CAD build for the part. Positions are in the model's coordinates, mm. A direction names the side the tool comes from. Round coordinates to 2 decimals unless told otherwise and drop trailing zeros. Order: outer loops, then holes, each group sorted by start corner. A loop starts at its lowest first (then second) coordinate and runs counter-clockwise, first axis right, second up. Notation, with made-up numbers: M 53,52.25 L 67,52.25 A31 ccw 67,91.25 Z; hole C 69,14 d8. An arc over 180 degrees is marked long. Put each result on its own line as item: value.
```python
from build123d import *

# Parameters (mm, degrees)
BOSS_EXTRUDE1_DEPTH = 6
SKETCH4_W           = 3
SKETCH4_H           = 3
CUT_EXTRUDE2_DEPTH  = 32
SKETCH5_R           = 1.75
CUT_EXTRUDE3_DEPTH  = 10


with BuildPart() as part:
    # Sketch1 → Boss-Extrude1 (new body)
    with BuildSketch(Plane(origin=(0, 0, 0), x_dir=(0, 1, 0), z_dir=(0, 0, 1))):
        with BuildLine():
            Line((-92.5, -9.5), (-94.5, -9.5))
            ThreePointArc((-94.5, -9.5), (-95.207106781, -9.792893219), (-95.5, -10.5))
            Line((-95.5, -10.5), (-95.5, -27.5))
            Line((-95.5, -27.5), (-95.5, -37.5))
            Line((-95.5, -37.5), (-99, -37.5))
            ThreePointArc((-99, -37.5), (-99.459572515, -37.196959649), (-99.362068966, -36.655172414))
            ThreePointArc((-99.362068966, -36.655172414), (-98.130927937, -34.737628825), (-97.7, -32.5))
            Line((-97.7, -32.5), (-97.7, -27.5))
            Line((-97.7, -27.5), (-99.2, -27.5))
            ThreePointArc((-99.2, -27.5), (-99.620181053, -27.271012699), (-99.655497604, -26.793791532))
            Line((-99.655497604, -26.793791532), (-98.212038328, -23.6053083))
            ThreePointArc((-98.212038328, -23.6053083), (-97.680035378, -21.993620083), (-97.5, -20.305972812))
            Line((-97.5, -20.305972812), (-97.5, -9.5))
            Line((-97.5, -9.5), (-97.5, 0.5))
            Line((-97.5, 0.5), (-92.5, 0.5))
            Line((-92.5, 0.5), (-92.5, 32.5))
            Line((-92.5, 32.5), (92.5, 32.5))
            Line((92.5, 32.5), (92.5, 0.5))
            Line((92.5, 0.5), (97.5, 0.5))
            Line((97.5, 0.5), (97.5, -9.5))
            Line((97.5, -9.5), (97.5, -20.305972812))
            ThreePointArc((97.5, -20.305972812), (97.680035378, -21.993620083), (98.212038328, -23.6053083))
            Line((98.212038328, -23.6053083), (99.655497604, -26.793791532))
            ThreePointArc((99.655497604, -26.793791532), (99.620181053, -27.271012699), (99.2, -27.5))
            Line((99.2, -27.5), (97.7, -27.5))
            Line((97.7, -27.5), (97.7, -32.5))
            ThreePointArc((97.7, -32.5), (98.130927937, -34.737628825), (99.362068966, -36.655172414))
            ThreePointArc((99.362068966, -36.655172414), (99.459572515, -37.196959649), (99, -37.5))
            Line((99, -37.5), (95.5, -37.5))
            Line((95.5, -37.5), (95.5, -27.5))
            Line((95.5, -27.5), (95.5, -10.5))
            ThreePointArc((95.5, -10.5), (95.207106781, -9.792893219), (94.5, -9.5))
            Line((94.5, -9.5), (92.5, -9.5))
            Line((92.5, -9.5), (92.5, -32.5))
            Line((92.5, -32.5), (-92.5, -32.5))
            Line((-92.5, -32.5), (-92.5, -9.5))
        make_face()
    extrude(amount=BOSS_EXTRUDE1_DEPTH)

    # Sketch4 → Cut-Extrude2 (cut)
    with BuildSketch(Plane(origin=(-32.5, 0, 0), x_dir=(0, -1, 0), z_dir=(-1, 0, 0))):
        with Locations((-91, 4.5)):
            Rectangle(SKETCH4_W, SKETCH4_H)
        with Locations((91, 4.5)):
            Rectangle(SKETCH4_W, SKETCH4_H)
    extrude(amount=-CUT_EXTRUDE2_DEPTH, mode=Mode.SUBTRACT)

    # Sketch5 → Cut-Extrude3 (cut)
    with BuildSketch(Plane.XY.offset(6)):
        with Locations((-27.94, 84.5)):
            Circle(SKETCH5_R)
        with Locations((-27.94, 15.92)):
            Circle(SKETCH5_R)
        with Locations((27.94, 15.92)):
            Circle(SKETCH5_R)
        with Locations((27.94, 84.5)):
            Circle(SKETCH5_R)
        with Locations((-27.94, -19.75)):
            Circle(SKETCH5_R)
        with Locations((-27.94, -85.5)):
            Circle(SKETCH5_R)
        with Locations((14.06, -85.5)):
            Circle(SKETCH5_R)
        with Locations((14.06, -19.75)):
            Circle(SKETCH5_R)
    extrude(amount=-CUT_EXTRUDE3_DEPTH, mode=Mode.SUBTRACT)


solid = part.part
```
Item 1: Band-saw the part on A-A on x = -27.94. Give the cut face in (y, z).
Answers below:
outline: M -92.5,0 L -87.25,0 L -87.25,6 L -89.5,6 L -89.5,3 L -92.5,3 Z; M -83.75,0 L -21.5,0 L -21.5,6 L -83.75,6 Z; M -18,0 L 14.17,0 L 14.17,6 L -18,6 Z; M 17.67,0 L 82.75,0 L 82.75,6 L 17.67,6 Z; M 86.25,0 L 92.5,0 L 92.5,3 L 89.5,3 L 89.5,6 L 86.25,6 Z
Item 2: Mould opens along Y. For faces 5 (the flat face through (2, 1, 6)), 6 (the flat face through (24, 95.5, 3)), 7 (the flat face through (25.222, -98.944, 2.958)) say: pulls with the +Y half, pulls with the -Y half, needs draft (parallel to the pull), parting line crosses it, or undercut.
Answers below:
face 5: needs draft
face 6: undercut
face 7: pulls with the -Y half
Item 3: Probe line 1 along Y through (x, z) = (27.94, 2.8); line 2 along Y through (x, z) = (-27.94, 3.75); line 3 along X through (y, z) = (-85.5, 4.5). List the from-to ranges inside material, lowest first. Write a range as [from, to].
Answers below:
line 1: [-97.7, -95.5], [-92.5, 14.17], [17.67, 82.75], [86.25, 92.5], [95.5, 97.7]
line 2: [-89.5, -87.25], [-83.75, -21.5], [-18, 14.17], [17.67, 82.75], [86.25, 89.5]
line 3: [-32.5, -29.69], [-26.19, 12.31], [15.81, 32.5]
Item 4: Band-saw the part on D-D on z = 3.95. State how many separate pieces and enclosed holes the cut face has, and give its area (3 significant figures).
Answers below:
separate pieces: 1
enclosed holes: 8
area: 12,000 mm²
Item 5: Band-saw the part on C-C on x = -2.5. Give the cut face in (y, z).
Answers below:
outline: M -92.5,0 L 92.5,0 L 92.5,3 L 89.5,3 L 89.5,6 L -89.5,6 L -89.5,3 L -92.5,3 Z
Item 6: Pin check, flat tips, straight feed: P1, Ø5.5, axis at x = -27.94, y = -85.5, coming from the +Z side; P2, Ø3, axis at y = -45, z = 4, coming from the +X side; P3, Ø1.8, axis at y = -94, z = 1.5, coming from the -X side; P4, Ø0.9, axis at x = -24, y = 91, coming from the +Z side. Stop position of each tip, or through.
Answers below:
P1: z = 6
P2: x = 32.5
P3: x = -0.5
P4: z = 3
Item 7: Band-saw the part on B-B on y = -85.5. Give the cut face in (x, z).
Answers below:
outline: M -32.5,0 L -29.69,0 L -29.69,6 L -32.5,6 Z; M -26.19,0 L 12.31,0 L 12.31,6 L -26.19,6 Z; M 15.81,0 L 32.5,0 L 32.5,6 L 15.81,6 Z
Item 8: Tool access for faces 1 (the flat face through (21, -92.5, 3)), 2 (the flat face through (30, 97.7, 3)), 3 (the flat face through (-32.5, -1, 3)), 4 (the flat face through (30, -97.7, 3)): list every direction of +Z, -Z, +X, -X, +Y, -Y with a clear straight run to the whole face (end or side of a thin tool).
Answers below:
face 1: +Z, -Z, +X
face 2: +Z, -Z, +Y
face 3: +Z, -Z, -X, +Y, -Y
face 4: +Z, -Z, -Y
